from build123d import *

# Parameters (mm, degrees)
ESBO_O1_R                = 3
RESSALTO_EXTRUS_O1_DEPTH = 20


with BuildPart() as part:
    # Esboço1 → Ressalto-extrusão1 (new body)
    with BuildSketch(Plane(origin=(0, 0, 0), x_dir=(1, 0, 0), z_dir=(0, 1, 0))):
        with BuildLine():
            Line((-7.056497116, 8.7), (-4, 8.7))
            Line((-4, 8.7), (-4, 10))
            Line((-4, 10), (-9.5, 10))
            ThreePointArc((-9.5, 10), (-9.853553391, 9.853553391), (-10, 9.5))
            Line((-10, 9.5), (-10, 4))
            Line((-10, 4), (-8.7, 4))
            Line((-8.7, 4), (-8.7, 7.056497116))
            ThreePointArc((-8.7, 7.056497116), (-8.51480503, 7.333660975), (-8.187867966, 7.26862915))
            Line((-8.187867966, 7.26862915), (-4.439339828, 3.520101013))
            ThreePointArc((-4.439339828, 3.520101013), (-4.114180701, 3.033465989), (-4, 2.459440841))
            Line((-4, 2.459440841), (-4, -2.459440841))
            ThreePointArc((-4, -2.459440841), (-4.114180701, -3.033465989), (-4.439339828, -3.520101013))
            Line((-4.439339828, -3.520101013), (-8.187867966, -7.26862915))
            ThreePointArc((-8.187867966, -7.26862915), (-8.51480503, -7.333660975), (-8.7, -7.056497116))
            Line((-8.7, -7.056497116), (-8.7, -4))
            Line((-8.7, -4), (-10, -4))
            Line((-10, -4), (-10, -9.5))
            ThreePointArc((-10, -9.5), (-9.853553391, -9.853553391), (-9.5, -10))
            Line((-9.5, -10), (-4, -10))
            Line((-4, -10), (-4, -8.7))
            Line((-4, -8.7), (-7.056497116, -8.7))
            ThreePointArc((-7.056497116, -8.7), (-7.333660975, -8.51480503), (-7.26862915, -8.187867966))
            Line((-7.26862915, -8.187867966), (-3.520101013, -4.439339828))
            ThreePointArc((-3.520101013, -4.439339828), (-3.033465989, -4.114180701), (-2.459440841, -4))
            Line((-2.459440841, -4), (2.459440841, -4))
            ThreePointArc((2.459440841, -4), (3.033465989, -4.114180701), (3.520101013, -4.439339828))
            Line((3.520101013, -4.439339828), (7.26862915, -8.187867966))
            ThreePointArc((7.26862915, -8.187867966), (7.333660975, -8.51480503), (7.056497116, -8.7))
            Line((7.056497116, -8.7), (4, -8.7))
            Line((4, -8.7), (4, -10))
            Line((4, -10), (9.5, -10))
            ThreePointArc((9.5, -10), (9.853553391, -9.853553391), (10, -9.5))
            Line((10, -9.5), (10, -4))
            Line((10, -4), (8.7, -4))
            Line((8.7, -4), (8.7, -7.056497116))
            ThreePointArc((8.7, -7.056497116), (8.51480503, -7.333660975), (8.187867966, -7.26862915))
            Line((8.187867966, -7.26862915), (4.439339828, -3.520101013))
            ThreePointArc((4.439339828, -3.520101013), (4.114180701, -3.033465989), (4, -2.459440841))
            Line((4, -2.459440841), (4, 2.459440841))
            ThreePointArc((4, 2.459440841), (4.114180701, 3.033465989), (4.439339828, 3.520101013))
            Line((4.439339828, 3.520101013), (8.187867966, 7.26862915))
            ThreePointArc((8.187867966, 7.26862915), (8.51480503, 7.333660975), (8.7, 7.056497116))
            Line((8.7, 7.056497116), (8.7, 4))
            Line((8.7, 4), (10, 4))
            Line((10, 4), (10, 9.5))
            ThreePointArc((10, 9.5), (9.853553391, 9.853553391), (9.5, 10))
            Line((9.5, 10), (4, 10))
            Line((4, 10), (4, 8.7))
            Line((4, 8.7), (7.056497116, 8.7))
            ThreePointArc((7.056497116, 8.7), (7.333660975, 8.51480503), (7.26862915, 8.187867966))
            Line((7.26862915, 8.187867966), (3.520101013, 4.439339828))
            ThreePointArc((3.520101013, 4.439339828), (3.033465989, 4.114180701), (2.459440841, 4))
            Line((2.459440841, 4), (-2.459440841, 4))
            ThreePointArc((-2.459440841, 4), (-3.033465989, 4.114180701), (-3.520101013, 4.439339828))
            Line((-3.520101013, 4.439339828), (-7.26862915, 8.187867966))
            ThreePointArc((-7.26862915, 8.187867966), (-7.333660975, 8.51480503), (-7.056497116, 8.7))
        make_face()
        Circle(ESBO_O1_R, mode=Mode.SUBTRACT)
    extrude(amount=RESSALTO_EXTRUS_O1_DEPTH)


solid = part.part
Design review of the part built by this model. Coordinates are the model's own, in mm. A direction names the side the tool comes from. Give positions to 0.01 mm unless a question says otherwise; leave off trailing zeros. Write each loop counter-clockwise with the first axis right and the second up, starting at its lowest first coordinate (ties: lowest second). Pieces come first, ordered by that corner, then holes. Notation, with made-up numbers: M 46,-21.5 L 86,-21.5 A20 ccw 86,7.5 Z; hole C 40.5,19.5 d1. An arc over 180 degrees is marked long. Answer as a JSON object with one key per item and string values. Group by question number.
1) For line 1 along X through (y, z) = (12.5, 0); line 2 along X through (y, z) = (18.25, 7.25), list the stretches that pass through material, from the lowest coordinate up.
2) We need section C-C (x = -6.25). Give the boundary of the cut face in (y, z).
3) We need section B-B (z = 0). Give the boundary of the cut face in (x, y).
4) We need section D-D (z = 6.5). Give the boundary of the cut face in (x, y), and give its area (3 significant figures).
5) Mouldability with a two-part tool opening along X and no side actions: class faces 1 (the face through (-4, 10, -9)), 2 (the face through (-10, 10, 7)), 3 (the face through (-9, 10, 4)) as released by +X, released by -X, zero draft, split by the parting line, or undercut.
6) Tool access review of faces 4 (the face through (-5.42, 9.86, 6.34)), 5 (the face through (-4.1, 9.9, -3)), 6 (the face through (9, 10, 4)), 7 (the face through (0, 10, -4)), 8 (the face through (3, 9.9, 4.1)): name each direction out of +Z, -Z, +X, -X, +Y, -Y from which nothing blocks a thin tool from reaching the whole face with its end or side.
7) Clearance check with flat-ended pins moving along their axes: pin 1 Ø3 at (x, y) = (-0.5, 10.5) entering from +Z; pin 2 Ø1.5 at (x, y) = (-0.5, 7.5) entering from -Z; pin 3 Ø1 at (y, z) = (6.5, 2) entering from +X. State where each tip first meets the part, or that it passes through.
8) We need section A-A (x = 0). Give the boundary of the cut face in (y, z), and give its area (3 significant figures).
Answer key:
{
 "1": {"line 1": "x = -4 to -3, 3 to 4", "line 2": "x = -10 to -8.63, -8.17 to -6.33, 6.33 to 8.17, 8.63 to 10"},
 "2": {"outline": "M 0,-10 L 20,-10 L 20,-8.7 L 0,-8.7 Z; M 0,-7.17 L 20,-7.17 L 20,-5.33 L 0,-5.33 Z; M 0,5.33 L 20,5.33 L 20,7.17 L 0,7.17 Z; M 0,8.7 L 20,8.7 L 20,10 L 0,10 Z"},
 "3": {"outline": "M -4,0 L -3,0 L -3,20 L -4,20 Z; M 3,0 L 4,0 L 4,20 L 3,20 Z"},
 "4": {"outline": "M -10,0 L -8.7,0 L -8.7,20 L -10,20 Z; M -7.42,0 L -5.58,0 L -5.58,20 L -7.42,20 Z; M 5.58,0 L 7.42,0 L 7.42,20 L 5.58,20 Z; M 8.7,0 L 10,0 L 10,20 L 8.7,20 Z", "area": "126 mm²"},
 "5": {"face 1": "undercut", "face 2": "released by -X", "face 3": "zero draft"},
 "6": {"face 4": "+Y, -Y", "face 5": "-X, +Y, -Y", "face 6": "+X, +Y, -Y", "face 7": "-Z, +Y, -Y", "face 8": "+Z, +Y, -Y"},
 "7": {"pin 1": "stops at z = 4", "pin 2": "stops at z = -4", "pin 3": "stops at x = 4"},
 "8": {"outline": "M 0,-4 L 20,-4 L 20,-3 L 0,-3 Z; M 0,3 L 20,3 L 20,4 L 0,4 Z", "area": "40.0 mm²"}
}
